For this review, take the finished solid that the model builds, in its own axes (mm). Face numbers are marked on the shaded views. A direction names the side the tool comes from. Coordinates: 2 decimals unless noted, no trailing zeros. Order: outer loops, then holes, each group sorted by start corner. A loop starts at its lowest first (then second) coordinate and runs counter-clockwise, first axis right, second up.
from build123d import *

# Parameters (mm, degrees)
BASENUTSKE_R  = 10.31875
BASENUT_DEPTH = 19.7104
SKETCH4_W     = 0.4064
SKETCH4_H     = 15.277682251


with BuildPart() as part:
    # BaseNutSke → BaseNut (new body)
    with BuildSketch(Plane.XY):
        Polygon((16.6624, 9.620041125), (16.6624, -9.620041125), (0, -19.240082251), (-16.6624, -9.620041125), (-16.6624, 9.620041125), (0, 19.240082251), align=None)
        Circle(BASENUTSKE_R, mode=Mode.SUBTRACT)
    extrude(amount=-BASENUT_DEPTH)

    # Sketch4 → Bearing-Face (revolve, cut)
    with BuildSketch(Plane(origin=(0, 0, 0), x_dir=(0, 0, -1), z_dir=(1, 0, 0))):
        with Locations((19.5072, 24.301241126)):
            Rectangle(SKETCH4_W, SKETCH4_H)
        Polygon((0, 16.6624), (-12.7, 16.6624), (-12.7, 31.940082251), (2.2225, 31.940082251), (2.2225, 19.240082251), align=None)
    revolve(axis=Axis((0, 0, 0), (0, 0, -1)), mode=Mode.SUBTRACT)

    # Sketch5 → EndChamfer (revolve, cut)
    with BuildSketch(Plane(origin=(0, 0, 0), x_dir=(0, 0, -1), z_dir=(1, 0, 0))):
        Polygon((19.685, 11.1125), (19.073631293, 10.239375), (19.7358, 10.239375), (19.7358, 11.1125), align=None)
        Polygon((-0.0508, 11.1125), (0, 11.1125), (0.611368707, 10.239375), (-0.0508, 10.239375), align=None)
    revolve(axis=Axis((0, 0, -25.037505729), (0, 0, -1)), mode=Mode.SUBTRACT)


solid = part.part
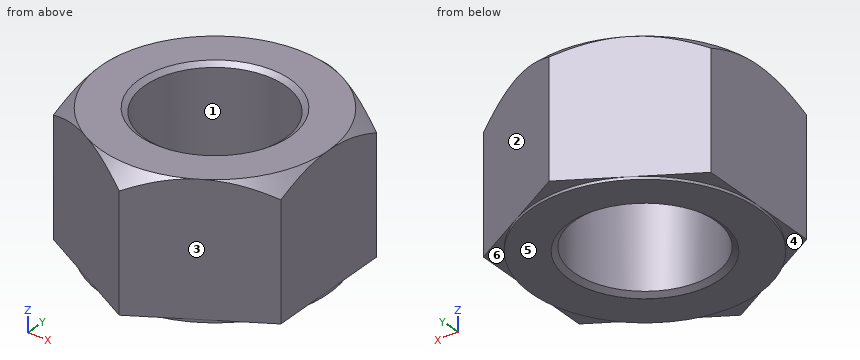
1. To check wall thickness, follow L1, parallel to X at y = 0, z = -12.75; L2, parallel to Y at x = 0, z = -12.5; L3, parallel to Y at x = -1, z = -5.25. State the ranges of each line that lie inside material, in increasing order.
Answer below:
L1: x = -16.66 to -10.32, 10.32 to 16.66
L2: y = -19.24 to -10.32, 10.32 to 19.24
L3: y = -18.66 to -10.27, 10.27 to 18.66
2. Take a section at A-A, the plane z = -9.25. Give the boundary of the cut face in (x, y).
Answer below:
outline: (-16.66, -9.62) - (0, -19.24) - (16.66, -9.62) - (16.66, 9.62) - (0, 19.24) - (-16.66, 9.62) - close; hole circle Ø20.64 at (0, 0)
3. Clearance check with flat-ended pins moving along their axes: pin 1 Ø5 at (x, z) = (12.5, -15.5) entering from +Y; pin 2 Ø6 at (x, z) = (-7.5, -8) entering from -Y; pin 3 Ø3 at (y, z) = (-14.5, -15.5) entering from -X. State where each tip first meets the part, or that it passes through.
Answer below:
pin 1: stops at y = 13.47
pin 2: stops at y = -16.64
pin 3: stops at x = -10.81
4. Machinability: for the marked faces 4, 5 and 6, which of the approach directions +Z, -Z, +X, -X, +Y, -Y give a long, thin tool a straight path to every point of the face, cutting with its end or side? Answer none if there is none.
Answer below:
face 4: -Z, -X, -Y
face 5: -Z, +X, -X, +Y, -Y
face 6: -Z, +X, +Y
5. The part is to be moulded in two halves that separate along Y. For the marked faces 1, 2 and 3, say which applies: +Y half, -Y half, draft (parallel to the pull), parting line (faces both ways), or undercut.
Answer below:
face 1: undercut
face 2: +Y half
face 3: -Y half
